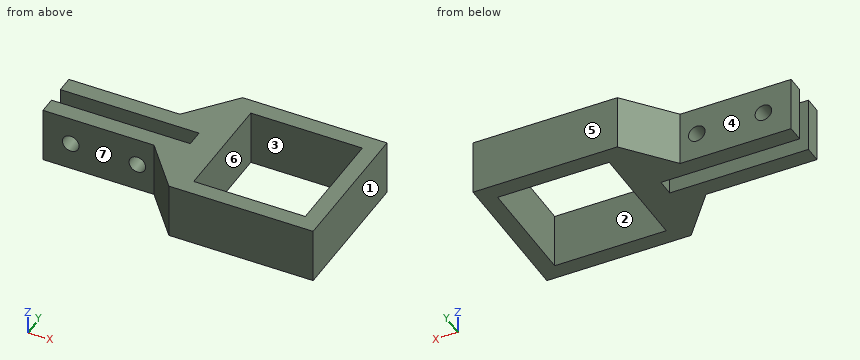
```python
from build123d import *

# Parameters (mm, degrees)
EXTRUDE_1_DEPTH     = 10
SKETCH_5_W          = 20.1
SKETCH_5_H          = 20.1
CUT_EXTRUDE_1_DEPTH = 30
SKETCH_7_R          = 1.5
CUT_EXTRUDE_5_DEPTH = 9.1


with BuildPart() as part:
    # 草图1 → 凸台-拉伸1 (new body)
    with BuildSketch(Plane.XY):
        Polygon((-27, 4.55), (-27, 1.55), (-2, 1.55), (-2, -1.55), (-27, -1.55), (-27, -4.55), (-7, -4.55), (0, -13), (26, -13), (26, 13), (0, 13), (-7, 4.55), align=None)
    extrude(amount=EXTRUDE_1_DEPTH)

    # 草图5 → 切除-拉伸1 (cut)
    with BuildSketch(Plane.XY.offset(10)):
        with Locations((13.05, -0.05)):
            Rectangle(SKETCH_5_W, SKETCH_5_H)
    extrude(amount=-CUT_EXTRUDE_1_DEPTH, mode=Mode.SUBTRACT)

    # 草图7 → 切除-拉伸5 (cut)
    with BuildSketch(Plane(origin=(0, 4.55, 0), x_dir=(1, 0, 0), z_dir=(0, 1, 0))):
        with Locations((-22, -5)):
            Circle(SKETCH_7_R)
        with Locations((-10, -5)):
            Circle(SKETCH_7_R)
    extrude(amount=-CUT_EXTRUDE_5_DEPTH, mode=Mode.SUBTRACT)


solid = part.part
```
Geometry check sheet. Reference: the model listing, model coordinates, mm. Face numbers are marked on the shaded views. A direction names the side the tool comes from. Give positions to 0.01 mm unless a question says otherwise; leave off trailing zeros. Write each loop counter-clockwise with the first axis right and the second up, starting at its lowest first coordinate (ties: lowest second). Pieces come first, ordered by that corner, then holes.
1) Material ranges on L1, parallel to X at y = -3.6, z = 5; L2, parallel to Y at x = 18, z = 5.5; L3, parallel to Z at x = -22, y = -3.2, recorded low to high.
2) Section check A-A, the plane x = -22. Record the boundary of the cut face in (y, z).
3) Access from +Z, -Z, +X, -X, +Y, -Y to the whole of each face (thin tool, end or side, straight path). Record for the marked faces 5, 6 and 7.
4) Section check B-B, the plane z = 5. State how many separate pieces and enclosed holes the cut face has, and give its area (3 significant figures).
5) Section check C-C, the plane y = 3.75. Record the boundary of the cut face in (x, z), and give its area (3 significant figures).
6) Gauge pin test, flat ends, axial feed: pin 1 (5 mm diameter, centred on x = -16, z = 3.5, fed in from +Y); pin 2 (3.5 mm diameter, centred on x = -10, z = 5, fed in from -Y); pin 3 (0.9 mm diameter, centred on y = 0.5, z = 5.5, fed in from -X). Record the tip position at first contact, or that the pin passes through.
7) Release check for a two-part mould opening along Y. For the marked faces 1, 2, 3 and 4 record: pulls with the +Y half, pulls with the -Y half, needs draft (parallel to the pull), parting line crosses it, or undercut.
8) Section check D-D, the plane y = 0.5. Record the boundary of the cut face in (x, z), and give its area (3 significant figures).
Computed:
1. L1: x = -27 to -23.5, -20.5 to -11.5, -8.5 to 3, 23.1 to 26
1. L2: y = -13 to -10.1, 10 to 13
1. L3: z = 0 to 3.5, 6.5 to 10
2. outline: (-4.55, 0) - (-1.55, 0) - (-1.55, 3.5) - (-4.55, 3.5) - close; (-4.55, 6.5) - (-1.55, 6.5) - (-1.55, 10) - (-4.55, 10) - close; (1.55, 0) - (4.55, 0) - (4.55, 3.5) - (1.55, 3.5) - close; (1.55, 6.5) - (4.55, 6.5) - (4.55, 10) - (1.55, 10) - close
3. face 5: +Z, -Z, +X, -X, +Y
3. face 6: +Z, -Z
3. face 7: +Z, -Z, -X, -Y
4. separate pieces: 5
4. enclosed holes: 1
4. area: 463 mm2
5. outline: (-27, 0) - (3, 0) - (3, 10) - (-27, 10) - close; (23.1, 0) - (26, 0) - (26, 10) - (23.1, 10) - close; hole circle Ø3 at (-22, 5); hole circle Ø3 at (-10, 5)
5. area: 315 mm2
6. pin 1: stops at y = 4.55
6. pin 2: stops at y = -4.55
6. pin 3: stops at x = -2
7. face 1: needs draft
7. face 2: undercut
7. face 3: undercut
7. face 4: pulls with the +Y half
8. outline: (-2, 0) - (3, 0) - (3, 10) - (-2, 10) - close; (23.1, 0) - (26, 0) - (26, 10) - (23.1, 10) - close
8. area: 79.0 mm2
